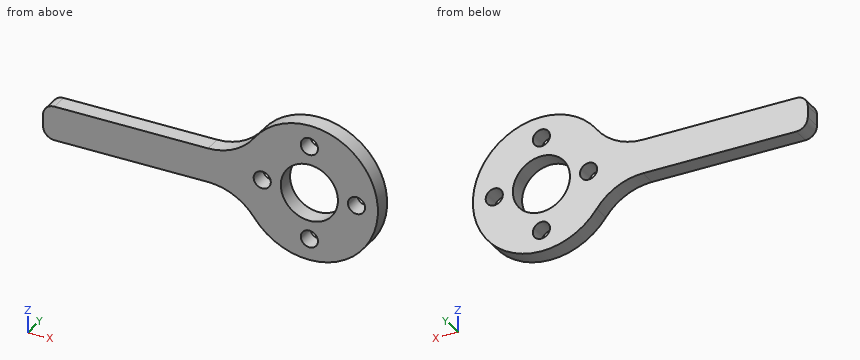
from build123d import *

# Parameters (mm, degrees)
SKETCH_1_R          = 5
EXTRUDE_1_DEPTH     = 3
SKETCH_2_R          = 1.5
CUT_EXTRUDE_1_DEPTH = 49.232007036
FILLET_1_R          = 2
FILLET_2_R          = 10


with BuildPart() as part:
    # 草图1 → 凸台-拉伸1 (new body)
    with BuildSketch(Plane(origin=(0, 0, 0), x_dir=(1, 0, 0), z_dir=(0, 1, 0))):
        with BuildLine():
            Line((-11.618950039, -3), (-46.618950039, -3))
            Line((-46.618950039, -3), (-46.618950039, 3))
            Line((-46.618950039, 3), (-11.618950039, 3))
            ThreePointArc((-11.618950039, 3), (12, 0), (-11.618950039, -3))
        make_face()
        with Locations(Location((0, 0, 0), (0, 0, 270))):
            Circle(SKETCH_1_R, mode=Mode.SUBTRACT)
    extrude(amount=EXTRUDE_1_DEPTH)

    # 草图2 → 切除-拉伸1 (cut, through all)
    with BuildSketch(Plane(origin=(0, 3, 0), x_dir=(1, 0, 0), z_dir=(0, 1, 0))):
        with Locations(Location((0, 8.25, 0), (0, 0, 270))):
            Circle(SKETCH_2_R)
        with Locations(Location((8.25, 0, 0), (0, 0, 270))):
            Circle(SKETCH_2_R)
        with Locations(Location((0, -8.25, 0), (0, 0, 270))):
            Circle(SKETCH_2_R)
        with Locations(Location((-8.25, 0, 0), (0, 0, 270))):
            Circle(SKETCH_2_R)
    extrude(amount=-CUT_EXTRUDE_1_DEPTH, mode=Mode.SUBTRACT)

    # 圆角1
    fillet_1_edges = [part.edges().sort_by_distance(p)[0] for p in [
        (-46.618950039, 1.5, 3),
        (-46.618950039, 1.5, -3),
    ]]
    fillet(fillet_1_edges, radius=FILLET_1_R)

    # 圆角2
    fillet_2_edges = [part.edges().sort_by_distance(p)[0] for p in [
        (-11.618950039, 1.5, 3),
        (-11.618950039, 1.5, -3),
    ]]
    fillet(fillet_2_edges, radius=FILLET_2_R)


solid = part.part
Verification items for the finished model (mm, model axes). Coordinates: 2 decimals unless noted, no trailing zeros. Order: outer loops, then holes, each group sorted by start corner. A loop starts at its lowest first (then second) coordinate and runs counter-clockwise, first axis right, second up. Notation, with made-up numbers: M 16.5,63.5 L 42.5,63.5 A20 cw 42.5,68.5 Z; hole C 51,8 d6. An arc over 180 degrees is marked long. One line per item, written item: value. Start each with the question number.
Item 1: Sectioned sample at D-D (z = -0.25). Enter the section's corners in (x, y), then the cut area to 3 significant figures.
Item 2: Sectioned sample at C-C (x = -8.25). Enter the section's corners in (y, z), then the cut area to 3 significant figures.
Item 3: Sectioned sample at B-B (z = 8.75). Enter the section's corners in (x, y).
Item 4: Sectioned sample at A-A (y = 0.55). Enter the section's corners in (x, z).
Item 5: Gauge pin test, flat ends, axial feed: pin 1 (1.5 mm diameter, centred on x = 2.5, y = 1, fed in from +Z); pin 2 (1.5 mm diameter, centred on x = -36, y = 1.5, fed in from -Z). Record the tip position at first contact, or that the pin passes through.
Item 6: Scan lines: probe 1 along X at (y, z) = (1.4, 8.25); probe 2 along X at (y, z) = (0.5, -0.75); probe 3 along Z at (x, y) = (-28, 2.4). Record each from-to range of solid material in increasing order.
Conclusion:
1. outline: M -46.62,0 L -9.73,0 L -9.73,3 L -46.62,3 Z; M -6.77,0 L -4.99,0 L -4.99,3 L -6.77,3 Z; M 4.99,0 L 6.77,0 L 6.77,3 L 4.99,3 Z; M 9.73,0 L 12,0 L 12,3 L 9.73,3 Z
1. area: 128 mm^2
2. outline: M 0,-8.71 L 3,-8.71 L 3,-1.5 L 0,-1.5 Z; M 0,1.5 L 3,1.5 L 3,8.71 L 0,8.71 Z
2. area: 43.3 mm^2
3. outline: M -8.21,0 L -1.41,0 L -1.41,3 L -8.21,3 Z; M 1.41,0 L 8.21,0 L 8.21,3 L 1.41,3 Z
4. outline: M -46.62,-1 A2 ccw -44.62,-3 L -17.75,-3 A10 cw -9.68,-7.09 A12 ccw long -9.68,7.09 A10 cw -17.75,3 L -44.62,3 A2 ccw -46.62,1 Z; hole C -8.25,0 d3; hole C 0,0 d10; hole C 0,-8.25 d3; hole C 0,8.25 d3; hole C 8.25,0 d3
5. pin 1: stops at z = 11.87
5. pin 2: stops at z = -3
6. probe 1: x = -8.71 to -1.5, 1.5 to 8.71
6. probe 2: x = -46.62 to -9.55, -6.95 to -4.94, 4.94 to 6.95, 9.55 to 11.98
6. probe 3: z = -3 to 3
